Input: part model. Units: mm. Frame: model coordinates. Face numbers are marked on the shaded views. A direction names the side the tool comes from. Give positions to 0.01 mm unless a question says otherwise; leave off trailing zeros. Write each loop counter-clockwise with the first axis right and the second up, starting at its lowest first coordinate (ties: lowest second). Pieces come first, ordered by that corner, then holes. Notation, with made-up numbers: (-2.5, -9.5) - (10.5, -9.5) arc R32 ccw to (10.5, 24.5) - close; hole circle Ø5 at (-39.75, 88). An arc over 180 degrees is marked (long way). Answer as CSV lines item,"result".
Autodesk Inventor part; units mm, degrees
ref_plane "Work Plane1" through (0, 8.1598, -7.7978) normal (0, 1, 0) x (-1, 0, 0)
ref_plane "YZ Plane" through (0, 0, 0) normal (1, 0, 0) x (0, 1, 0)
ref_plane "XZ Plane" through (0, 0, 0) normal (0, 1, 0) x (-1, 0, 0)
sketch "Sketch1" plane through (0, 0, 0) normal (0, 1, 0) x (-1, 0, 0)
  line L0 (0, 0) -> (15.5956, 0)
  line L1 (15.5956, 0) -> (15.5956, -15.5956)
  line L2 (15.5956, -15.5956) -> (0, -15.5956)
  line L3 (0, -15.5956) -> (0, 0)
  dimension "d0" = 15.5956
  dimension "d8" = 15.5956
extrude "Extrusion1" add sketch "Sketch1" along normal blind 9.6088
sketch "Sketch2" plane through (0, 9.6088, 0) normal (0, 1, 0) x (1, 0, 0)
  line L0 (0, 0) -> (-3.8989, 0) construction
  line L1 (-3.8989, 0) -> (-3.8989, 3.8989) construction
  line L2 (-3.8989, 3.8989) -> (0, 3.8989) construction
  line L3 (0, 3.8989) -> (0, 0) construction
  circle A0 centre (-3.8989, 3.8989) radius 2.4498
  dimension "d11" = 3.8989
  dimension "d12" = 3.8989
  dimension "d13" = 4.8997
extrude "Extrusion2" add sketch "Sketch2" along normal blind 1.9837
pattern_linear "Rectangular Pattern1" count 2 spacing 7.7978 along (0, 0, -1) count 2 spacing 7.7978 along (-1, 0, 0) of "Extrusion2"
shell "Shell1" thickness 1.4732 removed faces 1 at (-5.1985, 0, -5.1985)
sketch "Sketch3" plane through (-14.1224, 8.1356, -1.4732) normal (0, -1, 0) x (1, 0, 0)
  circle A0 centre (2.4257, -2.4257) radius 2.4498 construction
  circle A1 centre (10.2235, -10.2235) radius 2.4498 construction
  line L0 (2.4257, -2.4257) -> (10.2235, -10.2235) construction
  circle A2 centre (6.3246, -6.3246) radius 3.064
  circle A3 centre (6.3246, -6.3246) radius 2.4498
  point P0 (14.1224, 1.4732)
  dimension "d23" = 4.8997
extrude "Extrusion3" add sketch "Sketch3" along normal up to surface (8.1356 mm away)
sketch "Sketch4" plane through (0, 9.6088, 0) normal (0, 1, 0) x (1, 0, 0)
  circle A0 centre (-7.7978, 7.7978) radius 2.4498 construction
  circle A1 centre (-7.7978, 7.7978) radius 2.4498 construction
  line L0 (-9.0227, 5.6762) -> (-6.5729, 5.6762) construction
  line L1 (-6.5729, 5.6762) -> (-6.5729, 9.9194) construction
  line L2 (-6.5729, 9.9194) -> (-9.0227, 9.9194) construction
  line L3 (-9.0227, 9.9194) -> (-9.0227, 5.6762) construction
  line L4 (-9.0227, 5.6762) -> (-6.5729, 9.9194) construction
  line L5 (-6.5729, 5.6762) -> (-9.0227, 9.9194) construction
  line L6 (-9.9194, 9.0227) -> (-5.6762, 9.0227) construction
  line L7 (-5.6762, 9.0227) -> (-5.6762, 6.5729) construction
  line L8 (-5.6762, 6.5729) -> (-9.9194, 6.5729) construction
  line L9 (-9.9194, 6.5729) -> (-9.9194, 9.0227) construction
  line L10 (-9.9194, 9.0227) -> (-5.6762, 6.5729) construction
  line L11 (-5.6762, 9.0227) -> (-9.9194, 6.5729) construction
  line L12 (-9.0227, 9.0227) -> (-9.0227, 9.9194)
  line L13 (-6.5729, 9.9194) -> (-6.5729, 9.0227)
  line L14 (-6.5729, 9.0227) -> (-5.6762, 9.0227)
  line L15 (-5.6762, 6.5729) -> (-6.5729, 6.5729)
  line L16 (-6.5729, 6.5729) -> (-6.5729, 5.6762)
  line L17 (-9.0227, 5.6762) -> (-9.0227, 6.5729)
  line L18 (-9.0227, 6.5729) -> (-9.9194, 6.5729)
  line L19 (-9.9194, 9.0227) -> (-9.0227, 9.0227)
  arc A2 (-9.9194, 9.0227) -> (-9.9194, 6.5729) centre (-7.7978, 7.7978) ccw
  arc A3 (-6.5729, 9.9194) -> (-9.0227, 9.9194) centre (-7.7978, 7.7978) ccw
  arc A4 (-5.6762, 6.5729) -> (-5.6762, 9.0227) centre (-7.7978, 7.7978) ccw
  arc A5 (-9.0227, 5.6762) -> (-6.5729, 5.6762) centre (-7.7978, 7.7978) ccw
  point P0 (0, 0)
  dimension "d26" = 2.4498
  dimension "d27" = 2.4498
extrude "Extrusion4" cut sketch "Sketch4" against normal through all
sketch "Sketch5" plane through (0, 0, 0) normal (1, 0, 0) x (0, 0, -1)
  line L0 (0, 9.6088) -> (7.7978, 9.6088) construction
  line L1 (7.7978, 9.6088) -> (7.7978, 5.7099) construction
  line L2 (7.7978, 5.7099) -> (0, 5.7099) construction
  line L3 (0, 5.7099) -> (0, 9.6088) construction
  circle A0 centre (7.7978, 5.7099) radius 2.4498
  point P0 (0, 0)
  dimension "d30" = 7.7978
  dimension "d31" = 3.8989
  dimension "d32" = 4.8997
extrude "Extrusion5" add sketch "Sketch5" along normal blind 7.7978
sketch "Sketch6" plane through (7.7978, 5.7099, -7.7978) normal (1, 0, 0) x (0, 0, -1)
  circle A0 centre (0, 0) radius 2.4498 construction
  circle A1 centre (0, 0) radius 1.618
  point P0 (-7.7978, -5.7099)
  dimension "d35" = 3.236
extrude "Extrusion6" cut sketch "Sketch6" against normal blind 7.7978
sketch "Sketch7" plane through (-6.5729, 8.1356, -9.0227) normal (0, -1, 0) x (1, 0, 0)
  line L0 (-2.4498, 2.4498) -> (-2.4498, 3.3465) construction
  arc A0 (-2.4498, 3.3465) -> (-3.3465, 2.4498) centre (-1.2249, 1.2249) ccw construction
  line L1 (-3.3465, 2.4498) -> (-2.4498, 2.4498) construction
  line L2 (0, 2.4498) -> (0.8967, 2.4498) construction
  arc A1 (0.8967, 2.4498) -> (0, 3.3465) centre (-1.2249, 1.2249) ccw construction
  line L3 (0, 3.3465) -> (0, 2.4498) construction
  line L4 (0.8967, 0) -> (0, 0) construction
  line L5 (0, 0) -> (0, -0.8967) construction
  arc A2 (0, -0.8967) -> (0.8967, 0) centre (-1.2249, 1.2249) ccw construction
  line L6 (-2.4498, -0.8967) -> (-2.4498, 0) construction
  line L7 (-2.4498, 0) -> (-3.3465, 0) construction
  arc A3 (-3.3465, 0) -> (-2.4498, -0.8967) centre (-1.2249, 1.2249) ccw construction
  arc A4 (-2.4498, 3.3465) -> (-3.3465, 2.4498) centre (-1.2249, 1.2249) ccw
  arc A5 (0.8967, 0) -> (0.8967, 2.4498) centre (-1.2249, 1.2249) ccw
  arc A6 (0.8967, 2.4498) -> (0, 3.3465) centre (-1.2249, 1.2249) ccw
  arc A7 (-2.4498, -0.8967) -> (0, -0.8967) centre (-1.2249, 1.2249) ccw
  arc A8 (0, -0.8967) -> (0.8967, 0) centre (-1.2249, 1.2249) ccw
  arc A9 (-3.3465, 0) -> (-2.4498, -0.8967) centre (-1.2249, 1.2249) ccw
  line L8 (-2.4498, 3.3465) -> (-2.4498, 2.4498)
  line L9 (-2.4498, 2.4498) -> (-3.3465, 2.4498)
  line L10 (-2.4498, 2.4498) -> (-3.3465, 2.4498)
  line L11 (0, 2.4498) -> (0, 3.3465)
  line L12 (0, 3.3465) -> (0, 2.4498)
  line L13 (0, 2.4498) -> (0.8967, 2.4498)
  line L14 (0, 0) -> (0.8967, 0)
  line L15 (0.8967, 0) -> (0, 0)
  line L16 (0, 0) -> (0, -0.8967)
  line L17 (-2.4498, 0) -> (-2.4498, -0.8967)
  line L18 (-2.4498, -0.8967) -> (-2.4498, 0)
  arc A10 (-3.3465, 2.4498) -> (-3.3465, 0) centre (-1.2249, 1.2249) ccw
  line L19 (-2.4498, 0) -> (-3.3465, 0)
  point P0 (6.5729, 9.0227)
extrude "Extrusion7" add sketch "Sketch7" along normal up to surface (8.1356 mm away)
sketch "Sketch8" plane through (-7.7978, 0, -7.7978) normal (0, -1, 0) x (1, 0, 0)
  arc A0 (2.1216, -1.2249) -> (2.1216, 1.2249) centre (0, 0) ccw construction
  line L0 (2.1216, -1.2249) -> (1.2249, -1.2249) construction
  line L1 (1.2249, -1.2249) -> (1.2249, -2.1216) construction
  arc A1 (-1.2249, -2.1216) -> (1.2249, -2.1216) centre (0, 0) ccw construction
  line L2 (-1.2249, -2.1216) -> (-1.2249, -1.2249) construction
  line L3 (-1.2249, -1.2249) -> (-2.1216, -1.2249) construction
  arc A2 (-2.1216, 1.2249) -> (-2.1216, -1.2249) centre (0, 0) ccw construction
  line L4 (-2.1216, 1.2249) -> (-1.2249, 1.2249) construction
  line L5 (-1.2249, 1.2249) -> (-1.2249, 2.1216) construction
  arc A3 (1.2249, 2.1216) -> (-1.2249, 2.1216) centre (0, 0) ccw construction
  line L6 (1.2249, 2.1216) -> (1.2249, 1.2249) construction
  line L7 (1.2249, 1.2249) -> (2.1216, 1.2249) construction
  circle A4 centre (0, 0) radius 3.064 construction
  circle A5 centre (0, 0) radius 2.4498
  point P0 (7.7978, 7.7978)
extrude "Extrusion8" cut sketch "Sketch8" against normal blind 1.618
ref_plane "Work Plane1" through (0, 8.1598, -7.7978) normal (0, 1, 0) x (-1, 0, 0)
sketch "Sketch9" plane through (0, 8.1598, -7.7978) normal (0, 1, 0) x (-1, 0, 0)
  line L0 (-7.7978, 2.4498) -> (-7.7978, -2.4498) construction
  line L1 (-7.7978, 0) -> (-7.7978, 0.6125) construction
  line L2 (-7.7978, 0) -> (-7.1853, 0) construction
  line L3 (-7.7978, 0.6125) -> (-3.8989, 0.6125)
  line L4 (-3.8989, 0.6125) -> (-3.8989, -0.6125)
  line L5 (-3.8989, -0.6125) -> (-7.7978, -0.6125)
  line L6 (-7.7978, -0.6125) -> (-7.7978, 0.6125)
  point P0 (0, 7.7978)
  dimension "d42" = 0.6125
  dimension "d43" = 90
  dimension "d44" = 3.8989
  dimension "d45" = 1.2249
extrude "Extrusion9" cut sketch "Sketch9" against normal through all
equation "\"d0\" = 2 * d1"
equation "\"d8\" = 2 * d1"
equation "\"d9\" = d3"
equation "\"d11\" = 0.5 * d1"
equation "\"d12\" = 0.5 * d1"
equation "\"d13\" = d4"
equation "\"d14\" = d5"
equation "\"d18\" = d1"
equation "\"d21\" = d1"
equation "\"d22\" = d6"
equation "\"d23\" = d4"
equation "\"d24\" = d5"
equation "\"d26\" = 0.5 * d4"
equation "\"d27\" = 0.5 * d4"
equation "\"d28\" = d5"
equation "\"d30\" = d1"
equation "\"d31\" = 0.5 * d1"
equation "\"d32\" = d4"
equation "\"d33\" = d1"
equation "\"d35\" = d2"
equation "\"d36\" = d1"
equation "\"d40\" = 0.5 * d2"
equation "\"d42\" = 0.125 * d4"
equation "\"d44\" = 0.5 * d1"
equation "\"d45\" = 0.25 * d4"
equation "\"d46\" = 0.5 * d2"
equation "\"d1\" = 7.7978"
equation "\"d2\" = 3.23596"
equation "\"d3\" = 9.60882"
equation "\"d4\" = 4.89966"
equation "\"d5\" = 1.98374"
equation "\"d6\" = 1.4732"
equation "\"d7\" = 1.23952"
properties part number "2x2 tall things sticking out" material "ABS Plastic"
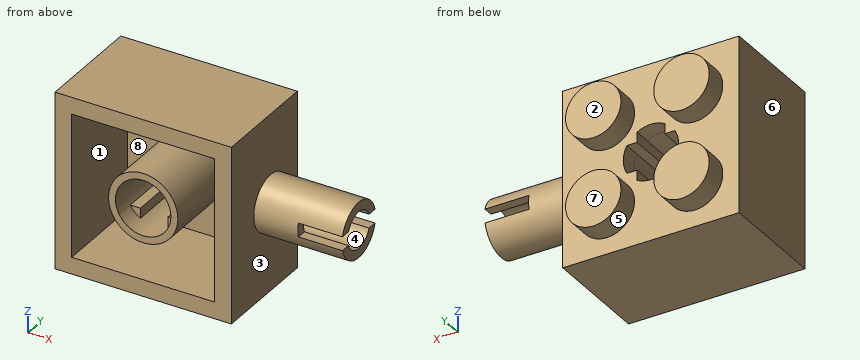
Item 1: Mould query, pull axis X, two halves, no side actions, for the marked faces 1, 2 and 3. Classes: +X half, -X half, draft (parallel to the pull), parting line (faces both ways), or undercut.
The answers:
face 1,"undercut"
face 2,"draft"
face 3,"+X half"
Item 2: Cut plane A-A on y = 6.25. Count the separate pieces of the cut face and the enclosed holes in it, plus the area to 3 significant figures.
The answers:
separate pieces,"2"
enclosed holes,"2"
area,"109 mm²"
Item 3: Contact query for flat-ended pins moving along their axis: pin 1 (5 mm diameter, centred on y = 8.5, z = -9.5, fed in from +X); pin 2 (1.6 mm diameter, centred on x = -3.9, z = -11.7, fed in from -Y); pin 3 (0.5 mm diameter, centred on y = 3.5, z = -7.5, fed in from +X). Output: stop coordinate, or through.
The answers:
pin 1,"x = 7.8"
pin 2,"y = 10.12"
pin 3,"x = 3.9"
Item 4: Ray query, line 1 (X direction, y = 8.5, z = -4); line 2 (X direction, y = 5.5, z = -8.25); line 3 (X direction, y = 3, z = -14). Return the intervals inside material, ascending. Write a range as from..to.
The answers:
line 1,"-15.6..-12.67, -10.73..-4.87, -2.93..0"
line 2,"-15.6..-14.12, -10.83..-10.21, -5.39..-4.77, -1.47..0"
line 3,"-15.6..-14.12, -1.47..0"
Item 5: Cut plane B-B on x = -6. Return the cut outline in (y, z), plus the area to 3 significant figures.
The answers:
outline,"(0, -15.6) - (9.61, -15.6) - (9.61, -12.96) - (11.59, -12.96) - (11.59, -10.44) - (9.61, -10.44) - (9.61, -9.02) - (1.62, -9.02) - (1.62, -9.46) - (0, -9.46) - (0, -10.28) - (8.14, -10.28) - (8.14, -14.12) - (0, -14.12) - close; (0, -6.13) - (1.62, -6.13) - (1.62, -6.57) - (9.61, -6.57) - (9.61, -5.16) - (11.59, -5.16) - (11.59, -2.64) - (9.61, -2.64) - (9.61, 0) - (0, 0) - (0, -1.47) - (8.14, -1.47) - (8.14, -5.32) - (0, -5.32) - close"
area,"72.4 mm²"
Item 6: Reachability of the marked faces 4, 5, 6, 7 and 8 from +Z, -Z, +X, -X, +Y, -Y: full face, straight path, thin tool, end or side. Return the list, or none.
The answers:
face 4,"+X"
face 5,"+Y"
face 6,"+Z, -Z, -X, +Y, -Y"
face 7,"+Z, -Z, +X, -X, +Y"
face 8,"-Y"
Item 7: Cut plane C-C on y = 2. Return the cut outline in (x, z), plus the area to 3 significant figures.
The answers:
outline,"(-15.6, -15.6) - (0, -15.6) - (0, 0) - (-15.6, 0) - close; circle Ø6.13 at (-7.8, -7.8); hole (-14.12, -14.12) - (-1.47, -14.12) - (-1.47, -1.47) - (-14.12, -1.47) - close; hole (-9.92, -9.02) - (-9.02, -9.02) - (-9.02, -9.92) arc R2.45 ccw to (-6.57, -9.92) - (-6.57, -9.02) - (-5.68, -9.02) arc R2.45 ccw to (-5.68, -6.57) - (-6.57, -6.57) - (-6.57, -5.68) arc R2.45 ccw to (-9.02, -5.68) - (-9.02, -6.57) - (-9.92, -6.57) arc R2.45 ccw to start"
area,"95.8 mm²"
Item 8: Cut plane D-D on z = -3.5. Return the cut outline in (x, y), plus the area to 3 significant figures.
The answers:
outline,"(-15.6, 0) - (-14.12, 0) - (-14.12, 8.14) - (-12.59, 8.14) - (-12.59, 10.12) - (-10.81, 10.12) - (-10.81, 8.14) - (-4.79, 8.14) - (-4.79, 10.12) - (-3.01, 10.12) - (-3.01, 8.14) - (-1.47, 8.14) - (-1.47, 0) - (0, 0) - (0, 9.61) - (-1.48, 9.61) - (-1.48, 11.59) - (-6.32, 11.59) - (-6.32, 9.61) - (-9.28, 9.61) - (-9.28, 11.59) - (-14.11, 11.59) - (-14.11, 9.61) - (-15.6, 9.61) - close"
area,"59.1 mm²"
